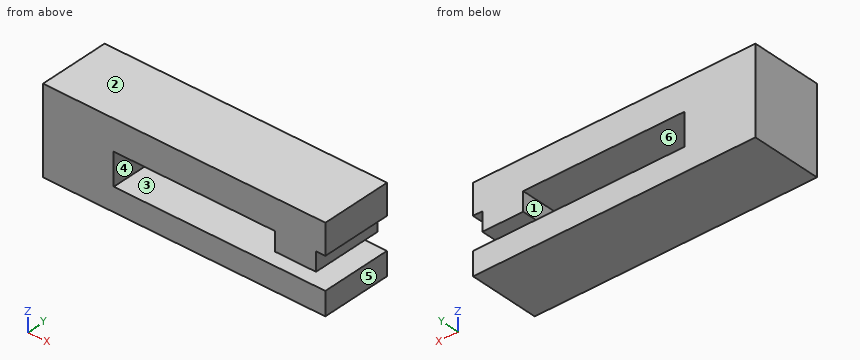
from build123d import *

# Parameters (mm, degrees)
F0_W     = 25.3896806389
F0_H     = 11.52669359
F0_W_2   = 14.6422572434
F0_H_2   = 6.7579634488
F1_DEPTH = 25.4


with BuildPart() as f1:
    # F0 (on Front) → F1 (new body)
    with BuildSketch(Plane.XZ):
        Polygon((52.3586980999, 30.7845659554), (-49.0107499063, 30.7845659554), (-49.0107499063, 19.8967363685), (-23.6210692674, 19.8967363685), (34.3374609947, 19.8967363685), (48.9797182381, 19.8967363685), (52.3586980999, 19.8967363685), align=None)
        with Locations((-36.3159095868, 14.1333895735)):
            Rectangle(F0_W, F0_H)
        Polygon((-23.6210692674, 8.3700427786), (-49.0107499063, 8.3700427786), (-49.0107499063, 0), (52.3202158511, 0), (52.3202158511, 8.3700427786), align=None)
        with Locations((41.6585896164, 16.5177546442)):
            Rectangle(F0_W_2, F0_H_2)
    extrude(amount=F1_DEPTH)


solid = f1.part
Can you work these out from the model? Positions are in its coordinate system, mm. Face numbers are marked on the shaded views. A direction names the side the tool comes from. Coordinates: 2 decimals unless noted, no trailing zeros. Loops run counter-clockwise (first coordinate to the right, second up) from the corner with the lowest first, then second, coordinate; pieces in that order, holes last. Notation, with made-up numbers: M -13,81.5 L -5,81.5 A15 ccw -5,97.5 Z; hole C 12,-7 d6. An arc over 180 degrees is marked long. Return JSON: item names as keys, results as strings. Group by question number.
Item 1: Imagine slicing it at D-D (z = 10.5). Please give me the cut outline in (x, y), and give its area (3 significant figures).
Item 2: I'm going to push flat-ended pins straight in: pin 1 Ø6 at (y, z) = (-10, 13.5) entering from +X; pin 2 Ø10 at (y, z) = (-7, 10.5) entering from +X. Where does each tip first touch, or does it pass through?
Item 3: Imagine slicing it at C-C (y = -16). Please give me the cut outline in (x, z).
Item 4: Imagine slicing it at A-A (x = 43.5). Please give me the cut outline in (y, z).
Item 5: If I drill on L1, parallel to Z at x = 12, y = -13; L2, parallel to Z at x = 39.5, y = -19.25; L3, parallel to X at y = -12.5, z = 18.5, over which ranges is the centre line in solid material (lowest first)? Write a range as from..to.
Item 6: Imagine slicing it at B-B (z = 18). Please give me the cut outline in (x, y), and give its area (3 significant figures).
Item 7: On a 3-axis mill with a long thin cutter (end or side, diameter ignored), from which of +Z, -Z, +X, -X, +Y, -Y can I reach the whole of each face in a straight line? I mean the marked faces 1 and 2. Say none if no direction works.
Item 8: Thinking about a two-plate mould opening in X: for the marked faces 3, 4, 5 and 6, which applies, released by +X, released by -X, zero draft, split by the parting line, or undercut?
Verdict:
{
 "1": {"outline": "M -49.01,-25.4 L -23.62,-25.4 L -23.62,0 L -49.01,0 Z", "area": "645 mm^2"},
 "2": {"pin 1": "stops at x = 48.98", "pin 2": "stops at x = 52.32"},
 "3": {"outline": "M -49.01,0 L 52.32,0 L 52.32,8.37 L -23.62,8.37 L -23.62,19.9 L 34.34,19.9 L 34.34,13.14 L 48.98,13.14 L 48.98,19.9 L 52.36,19.9 L 52.36,30.78 L -49.01,30.78 Z"},
 "4": {"outline": "M -25.4,0 L 0,0 L 0,8.37 L -25.4,8.37 Z; M -25.4,13.14 L 0,13.14 L 0,30.78 L -25.4,30.78 Z"},
 "5": {"L1": "z = 0..8.37, 19.9..30.78", "L2": "z = 0..8.37, 13.14..30.78", "L3": "x = -49.01..-23.62, 34.34..48.98"},
 "6": {"outline": "M -49.01,-25.4 L -23.62,-25.4 L -23.62,0 L -49.01,0 Z; M 34.34,-25.4 L 48.98,-25.4 L 48.98,0 L 34.34,0 Z", "area": "1,020 mm^2"},
 "7": {"face 1": "+Y, -Y", "face 2": "+Z, +X, -X, +Y, -Y"},
 "8": {"face 3": "zero draft", "face 4": "undercut", "face 5": "released by +X", "face 6": "undercut"}
}
